Could you check a few things on this model? Use its own coordinates, in mm. A direction names the side the tool comes from. Give positions to 0.01 mm unless a question says otherwise; leave off trailing zeros. Write each loop counter-clockwise with the first axis right and the second up, starting at its lowest first coordinate (ties: lowest second). Pieces come first, ordered by that corner, then holes. Notation, with made-up numbers: (-11.5, -7.5) - (11.5, -7.5) arc R13 ccw to (11.5, 3.5) - close; hole circle Ø5 at (40, 6.5). An arc over 180 degrees is marked (long way). Answer in a Markdown table with one row per item.
from build123d import *

# Parameters (mm, degrees)
CROQUIS1_W                = 114
CROQUIS1_H                = 202
SALIENTE_EXTRUIR1_DEPTH   = 30.5
CROQUIS2_W                = 2
CROQUIS2_H                = 18
CORTAR_EXTRUIR1_DEPTH     = 62
MATRIZL1_COUNT            = 9
MATRIZL1_PITCH            = 22
SIMETR_A1_COPY_1_SKETCH_W = 2
SIMETR_A1_COPY_1_SKETCH_H = 18
SIMETR_A1_COPY_1_DEPTH    = 62
SIMETR_A1_COPY_2_SKETCH_W = 2
SIMETR_A1_COPY_2_SKETCH_H = 18
SIMETR_A1_COPY_2_DEPTH    = 62
SIMETR_A1_COPY_3_SKETCH_W = 2
SIMETR_A1_COPY_3_SKETCH_H = 18
SIMETR_A1_COPY_3_DEPTH    = 62
SIMETR_A1_COPY_4_SKETCH_W = 2
SIMETR_A1_COPY_4_SKETCH_H = 18
SIMETR_A1_COPY_4_DEPTH    = 62
SIMETR_A1_COPY_5_SKETCH_W = 2
SIMETR_A1_COPY_5_SKETCH_H = 18
SIMETR_A1_COPY_5_DEPTH    = 62
SIMETR_A1_COPY_6_SKETCH_W = 2
SIMETR_A1_COPY_6_SKETCH_H = 18
SIMETR_A1_COPY_6_DEPTH    = 62
SIMETR_A1_COPY_7_SKETCH_W = 2
SIMETR_A1_COPY_7_SKETCH_H = 18
SIMETR_A1_COPY_7_DEPTH    = 62
SIMETR_A1_COPY_8_SKETCH_W = 2
SIMETR_A1_COPY_8_SKETCH_H = 18
SIMETR_A1_COPY_8_DEPTH    = 62
CROQUIS3_W                = 18
CROQUIS3_H                = 2
CORTAR_EXTRUIR2_DEPTH     = 203
CROQUIS4_W                = 102
CROQUIS4_H                = 49
CORTAR_EXTRUIR3_DEPTH     = 4
CROQUIS5_R                = 9
SALIENTE_EXTRUIR2_DEPTH   = 5
CROQUIS6_R                = 3
CORTAR_EXTRUIR4_DEPTH     = 10


with BuildPart() as part:
    # Croquis1 → Saliente-Extruir1 (new body, symmetric)
    with BuildSketch(Plane.XY):
        Rectangle(CROQUIS1_W, CROQUIS1_H)
    extrude(amount=SALIENTE_EXTRUIR1_DEPTH, both=True)

    # Croquis2 → Cortar-Extruir1 (cut, through all)
    with BuildSketch(Plane.XY.offset(30.5)):
        with Locations((56, 88)):
            Rectangle(CROQUIS2_W, CROQUIS2_H)
    cortar_extruir1 = extrude(amount=-CORTAR_EXTRUIR1_DEPTH, mode=Mode.SUBTRACT)

    # MatrizL1: Cortar-Extruir1 ×9
    with Locations(*[(0, -i * MATRIZL1_PITCH, 0) for i in range(1, MATRIZL1_COUNT)]):
        add(cortar_extruir1, mode=Mode.SUBTRACT)

    # Simetría1: Cortar-Extruir1 across plane
    add(cortar_extruir1.mirror(Plane(origin=(0, 0, 0), x_dir=(0, 0, 1), z_dir=(1, 0, 0))), mode=Mode.SUBTRACT)

    # Simetría1 copy 1 sketch → Simetría1 copy 1 (cut, through all)
    with BuildSketch(Plane(origin=(0, -22, 30.5), x_dir=(-1, 0, 0), z_dir=(0, 0, 1))):
        with Locations((56, -88)):
            Rectangle(SIMETR_A1_COPY_1_SKETCH_W, SIMETR_A1_COPY_1_SKETCH_H)
    extrude(amount=-SIMETR_A1_COPY_1_DEPTH, mode=Mode.SUBTRACT)

    # Simetría1 copy 2 sketch → Simetría1 copy 2 (cut, through all)
    with BuildSketch(Plane(origin=(0, -44, 30.5), x_dir=(-1, 0, 0), z_dir=(0, 0, 1))):
        with Locations((56, -88)):
            Rectangle(SIMETR_A1_COPY_2_SKETCH_W, SIMETR_A1_COPY_2_SKETCH_H)
    extrude(amount=-SIMETR_A1_COPY_2_DEPTH, mode=Mode.SUBTRACT)

    # Simetría1 copy 3 sketch → Simetría1 copy 3 (cut, through all)
    with BuildSketch(Plane(origin=(0, -66, 30.5), x_dir=(-1, 0, 0), z_dir=(0, 0, 1))):
        with Locations((56, -88)):
            Rectangle(SIMETR_A1_COPY_3_SKETCH_W, SIMETR_A1_COPY_3_SKETCH_H)
    extrude(amount=-SIMETR_A1_COPY_3_DEPTH, mode=Mode.SUBTRACT)

    # Simetría1 copy 4 sketch → Simetría1 copy 4 (cut, through all)
    with BuildSketch(Plane(origin=(0, -88, 30.5), x_dir=(-1, 0, 0), z_dir=(0, 0, 1))):
        with Locations((56, -88)):
            Rectangle(SIMETR_A1_COPY_4_SKETCH_W, SIMETR_A1_COPY_4_SKETCH_H)
    extrude(amount=-SIMETR_A1_COPY_4_DEPTH, mode=Mode.SUBTRACT)

    # Simetría1 copy 5 sketch → Simetría1 copy 5 (cut, through all)
    with BuildSketch(Plane(origin=(0, -110, 30.5), x_dir=(-1, 0, 0), z_dir=(0, 0, 1))):
        with Locations((56, -88)):
            Rectangle(SIMETR_A1_COPY_5_SKETCH_W, SIMETR_A1_COPY_5_SKETCH_H)
    extrude(amount=-SIMETR_A1_COPY_5_DEPTH, mode=Mode.SUBTRACT)

    # Simetría1 copy 6 sketch → Simetría1 copy 6 (cut, through all)
    with BuildSketch(Plane(origin=(0, -132, 30.5), x_dir=(-1, 0, 0), z_dir=(0, 0, 1))):
        with Locations((56, -88)):
            Rectangle(SIMETR_A1_COPY_6_SKETCH_W, SIMETR_A1_COPY_6_SKETCH_H)
    extrude(amount=-SIMETR_A1_COPY_6_DEPTH, mode=Mode.SUBTRACT)

    # Simetría1 copy 7 sketch → Simetría1 copy 7 (cut, through all)
    with BuildSketch(Plane(origin=(0, -154, 30.5), x_dir=(-1, 0, 0), z_dir=(0, 0, 1))):
        with Locations((56, -88)):
            Rectangle(SIMETR_A1_COPY_7_SKETCH_W, SIMETR_A1_COPY_7_SKETCH_H)
    extrude(amount=-SIMETR_A1_COPY_7_DEPTH, mode=Mode.SUBTRACT)

    # Simetría1 copy 8 sketch → Simetría1 copy 8 (cut, through all)
    with BuildSketch(Plane(origin=(0, -176, 30.5), x_dir=(-1, 0, 0), z_dir=(0, 0, 1))):
        with Locations((56, -88)):
            Rectangle(SIMETR_A1_COPY_8_SKETCH_W, SIMETR_A1_COPY_8_SKETCH_H)
    extrude(amount=-SIMETR_A1_COPY_8_DEPTH, mode=Mode.SUBTRACT)

    # Croquis3 → Cortar-Extruir2 (cut, through all)
    with BuildSketch(Plane(origin=(0, 101, 0), x_dir=(1, 0, 0), z_dir=(0, 1, 0))):
        with Locations((0, 29.5)):
            Rectangle(CROQUIS3_W, CROQUIS3_H)
        with Locations((21, 29.5)):
            Rectangle(CROQUIS3_W, CROQUIS3_H)
        with Locations((42, 29.5)):
            Rectangle(CROQUIS3_W, CROQUIS3_H)
        with Locations((-42, 29.5)):
            Rectangle(CROQUIS3_W, CROQUIS3_H)
        with Locations((-21, 29.5)):
            Rectangle(CROQUIS3_W, CROQUIS3_H)
    cortar_extruir2 = extrude(amount=-CORTAR_EXTRUIR2_DEPTH, mode=Mode.SUBTRACT)

    # Simetría2: Cortar-Extruir2 across plane
    add(cortar_extruir2.mirror(Plane.XY), mode=Mode.SUBTRACT)

    # Croquis4 → Cortar-Extruir3 (cut)
    with BuildSketch(Plane(origin=(0, 101, 0), x_dir=(1, 0, 0), z_dir=(0, 1, 0))):
        Rectangle(CROQUIS4_W, CROQUIS4_H)
    extrude(amount=-CORTAR_EXTRUIR3_DEPTH, mode=Mode.SUBTRACT)

    # Croquis5 → Saliente-Extruir2 (add)
    with BuildSketch(Plane(origin=(0, 97, 0), x_dir=(1, 0, 0), z_dir=(0, 1, 0))):
        with Locations((32.053240518, 0)):
            Circle(CROQUIS5_R)
    saliente_extruir2 = extrude(amount=SALIENTE_EXTRUIR2_DEPTH)

    # Croquis6 → Cortar-Extruir4 (cut)
    with BuildSketch(Plane(origin=(0, 102, 0), x_dir=(1, 0, 0), z_dir=(0, 1, 0))):
        with Locations((32.053240518, 0)):
            Circle(CROQUIS6_R)
    cortar_extruir4 = extrude(amount=-CORTAR_EXTRUIR4_DEPTH, mode=Mode.SUBTRACT)

    # Simetría4: Saliente-Extruir2, Cortar-Extruir4 across plane
    add(saliente_extruir2.mirror(Plane(origin=(0, 0, 0), x_dir=(0, 0, 1), z_dir=(1, 0, 0))))
    add(cortar_extruir4.mirror(Plane(origin=(0, 0, 0), x_dir=(0, 0, 1), z_dir=(1, 0, 0))), mode=Mode.SUBTRACT)


solid = part.part
1) We'd pull the mould along X, two halves only. Please class faces 1 (the face through (51, 99, 0)), 2 (the face through (-57, -77, 0)), 3 (the face through (55, -44, 0)): +X half, -X half, draft (parallel to the pull), parting line (faces both ways), or undercut.
Check values:
| item | result |
|---|---|
| face 1 | undercut |
| face 2 | -X half |
| face 3 | +X half |
2) If I drill on line 1 (X direction, y = 99, z = 0); line 2 (X direction, y = 96.5, z = 0); line 3 (Y direction, x = 13.5, z = 10.5), over which ranges is the centre line in solid material (lowest first)?
Check values:
| item | result |
|---|---|
| line 1 | x = -57 to -51, -41.05 to -35.05, -29.05 to -23.05, 23.05 to 29.05, 35.05 to 41.05, 51 to 57 |
| line 2 | x = -55 to -35.05, -29.05 to 29.05, 35.05 to 55 |
| line 3 | y = -101 to 97 |
3) Imagine slicing it at A-A (x = 44.5). List the corners of the cut face in (y, z) for me, then the cut area to 3 significant figures.
Check values:
| item | result |
|---|---|
| outline | (-101, -28.5) - (101, -28.5) - (101, -24.5) - (97, -24.5) - (97, 24.5) - (101, 24.5) - (101, 28.5) - (-101, 28.5) - close |
| area | 11,300 mm2 |
4) On a 3-axis mill with a long thin cutter (end or side, diameter ignored), from which of +Z, -Z, +X, -X, +Y, -Y can I reach the whole of each face in a straight line? I mean faces 4 (the face through (55, -88, 0)), 5 (the face through (-1, 99, 24.5)), 6 (the face through (-55, -22, 0)), 7 (the face through (42, 1, -28.5)), 8 (the face through (57, -99, 0)). Say none if no direction works.
Check values:
| item | result |
|---|---|
| face 4 | +Z, -Z, +X |
| face 5 | +Y |
| face 6 | +Z, -Z, -X |
| face 7 | -Z, +Y, -Y |
| face 8 | +Z, -Z, +X, +Y, -Y |
5) Will these pins go through, and if not, where does the flat tip stop? P1, Ø5.5, axis at y = -4, z = -1, coming from the +X side; P2, Ø1.5, axis at x = 45.5, z = 10.5, coming from the +Y side; P3, Ø0.6, axis at y = 8.5, z = -29.5, coming from the -X side.
Check values:
| item | result |
|---|---|
| P1 | stops at x = 55 |
| P2 | stops at y = 97 |
| P3 | stops at x = -55 |
